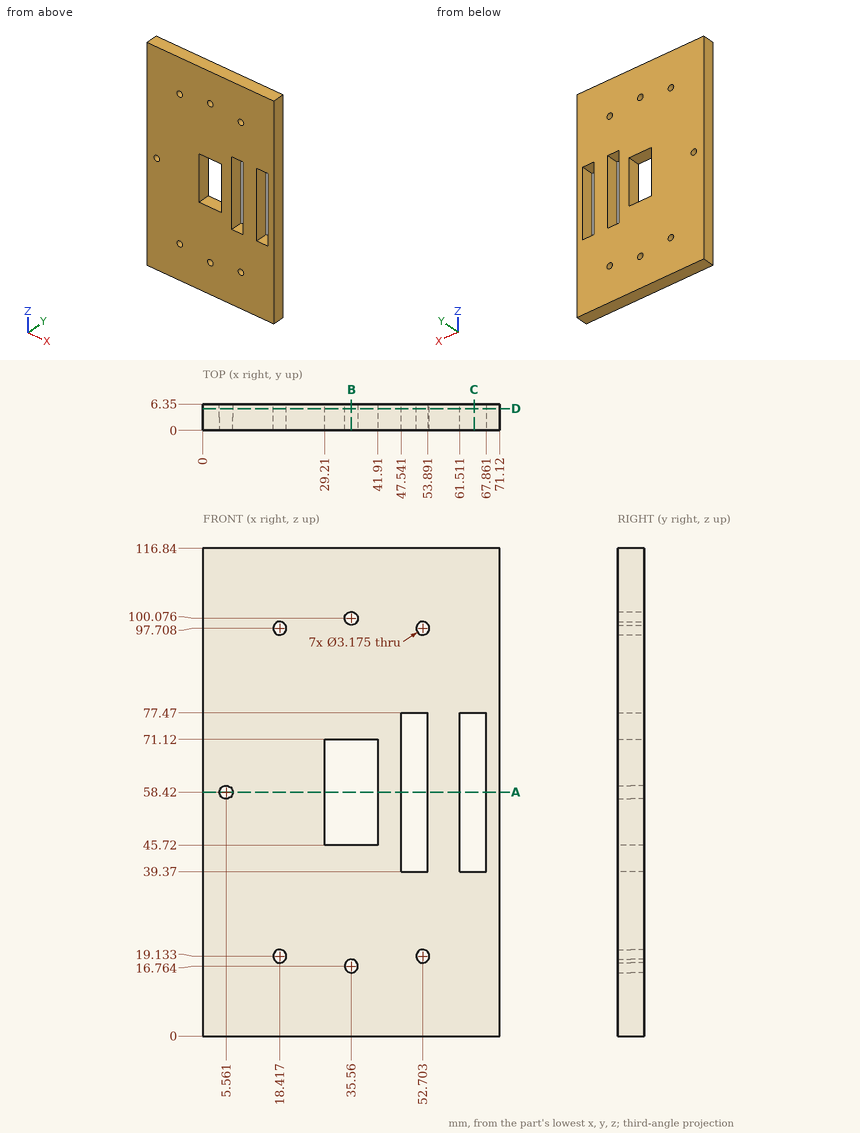
Print and shaded views of the part. All mm, measured from the part's lowest x, y and z. Round coordinates to 2 decimals unless told otherwise and drop trailing zeros. Write each loop counter-clockwise with the first axis right and the second up, starting at its lowest first coordinate (ties: lowest second). Pieces come first, ordered by that corner, then holes. Notation, with made-up numbers: (69.5, -22.5) - (120.5, -22.5) arc R17 ccw to (120.5, -9.5) - close; hole circle Ø2 at (-20.5, 87). An arc over 180 degrees is marked (long way). Use CSV: the item, a comma, the result in double quotes. Start each with the question number.
Item 1: Band-saw the part on A-A (z = 58.42). Write the cut outline in (x, y), and give its area (3 significant figures).
Item 2: Drill centre lines: L1, parallel to X at y = 3.5, z = 50; L2, parallel to Z at x = 29.5, y = 2.5; L3, parallel to Z at x = 35.56, y = 5.05. Where is each one in solid material? Low to high. Write a range as [from, to].
Item 3: Band-saw the part on B-B (x = 35.56). Write the cut outline in (y, z).
Item 4: Band-saw the part on C-C (x = 65). Write the cut outline in (y, z), and give its area (3 significant figures).
Item 5: Pin check, flat tip, straight feed: P1, Ø3, axis at x = 51, y = 3, coming from the -Z side. Stop position of the tip, or through.
Item 6: Band-saw the part on D-D (y = 5.25). State how many separate pieces and enclosed holes the cut face has, and give its area (3 significant figures).
Checked values:
1,outline,"(0, 0) - (3.97, 0) - (3.97, 6.35) - (0, 6.35) - close; (7.15, 0) - (29.21, 0) - (29.21, 6.35) - (7.15, 6.35) - close; (41.91, 0) - (47.54, 0) - (47.54, 6.35) - (41.91, 6.35) - close; (53.89, 0) - (61.51, 0) - (61.51, 6.35) - (53.89, 6.35) - close; (67.86, 0) - (71.12, 0) - (71.12, 6.35) - (67.86, 6.35) - close"
1,area,"270 mm²"
2,L1,"x = [0, 29.21], [41.91, 47.54], [53.89, 61.51], [67.86, 71.12]"
2,L2,"z = [0, 45.72], [71.12, 116.84]"
2,L3,"z = [0, 15.18], [18.35, 45.72], [71.12, 98.49], [101.66, 116.84]"
3,outline,"(0, 0) - (6.35, 0) - (6.35, 15.18) - (0, 15.18) - close; (0, 18.35) - (6.35, 18.35) - (6.35, 45.72) - (0, 45.72) - close; (0, 71.12) - (6.35, 71.12) - (6.35, 98.49) - (0, 98.49) - close; (0, 101.66) - (6.35, 101.66) - (6.35, 116.84) - (0, 116.84) - close"
4,outline,"(0, 0) - (6.35, 0) - (6.35, 39.37) - (0, 39.37) - close; (0, 77.47) - (6.35, 77.47) - (6.35, 116.84) - (0, 116.84) - close"
4,area,"500 mm²"
5,P1,"stops at z = 0"
6,separate pieces,"1"
6,enclosed holes,"10"
6,area,"7,450 mm²"
